Geometry: final body of the model. Coordinates: model frame, mm. Face numbers are marked on the shaded views. A direction names the side the tool comes from. Coordinates: 2 decimals unless noted, no trailing zeros. Use CSV: the item, a comma, the result in double quotes. Start each with the question number.
1. Set-up query: the marked faces 1, 2 and 3. Return all of +Z, -Z, +X, -X, +Y, -Y with unobstructed straight access to the full face (end or side cutting, diameter ignored); none if empty.
2. Material intervals for line 1 (X direction, y = -4.5, z = 0); line 2 (Z direction, x = 14.2, y = -2.75); line 3 (Y direction, x = -9, z = 9.5), sorted ascending.
3. First-contact query: P1, Ø1.6, axis at x = 1, y = 2, coming from the +Z side; P2, Ø2.5, axis at x = -4.5, y = 2, coming from the -Z side; P3, Ø1, axis at y = 1, z = 4, coming from the +X side; P4, Ø3, axis at x = -12.5, y = 8.5, coming from the -Z side. Flat tips, straight axial feed; report the tip coordinate or a pass-through.
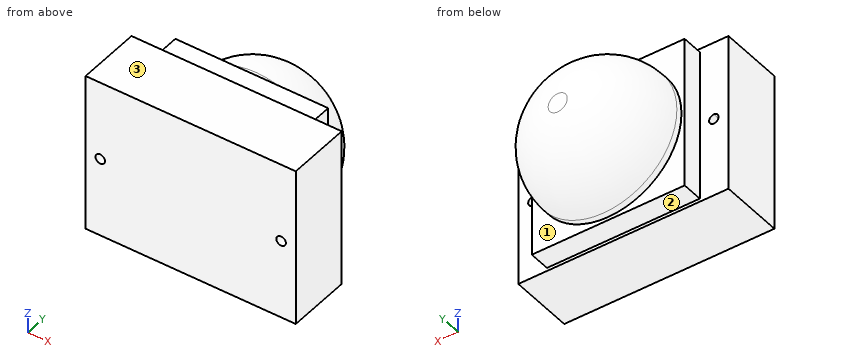
from build123d import *

# Parameters (mm, degrees)
F0_W     = 24
F0_H     = 24
F1_DEPTH = 10
F2_DEPTH = 3.3
F3_R     = 11.5
F4_DEPTH = 11
F5_R     = 10
F6_DEPTH = 10


with BuildPart() as f1:
    # F0 (on Front) → F1 (new body)
    with BuildSketch(Plane.XZ):
        with BuildLine():
            ThreePointArc((14.95, 0), (14.73033, 0.53033), (14.2, 0.75))
            ThreePointArc((14.2, 0.75), (13.66967, -0.53033), (14.95, 0))
        make_face()
        with BuildLine():
            ThreePointArc((-13.45, 0), (-13.66967, 0.53033), (-14.2, 0.75))
            ThreePointArc((-14.2, 0.75), (-14.73033, -0.53033), (-13.45, 0))
        make_face()
        Polygon((-16.5, -12.5), (16.5, -12.5), (16.5, 12.5), (14.2, 12.5), (-14.2, 12.5), (-16.5, 12.5), align=None)
        with BuildLine():
            ThreePointArc((-13.45, 0), (-14.73033, -0.53033), (-14.2, 0.75))
            ThreePointArc((-14.2, 0.75), (-13.66967, 0.53033), (-13.45, 0))
        make_face(mode=Mode.SUBTRACT)
        Rectangle(F0_W, F0_H, mode=Mode.SUBTRACT)
        with BuildLine():
            ThreePointArc((14.95, 0), (13.66967, -0.53033), (14.2, 0.75))
            ThreePointArc((14.2, 0.75), (14.73033, 0.53033), (14.95, 0))
        make_face(mode=Mode.SUBTRACT)
        Rectangle(F0_W, F0_H)
    extrude(amount=F1_DEPTH)

    # F0 (on Front) → F2 (join)
    with BuildSketch(Plane.XZ):
        Rectangle(F0_W, F0_H)
    extrude(amount=-F2_DEPTH)

    # F3 (on face) → F4 (join)
    with BuildSketch(Plane(origin=(0, 3.3, 0), x_dir=(-1, 0, 0), z_dir=(0, 1, 0))):
        Circle(F3_R)
    extrude(amount=F4_DEPTH)

    # F5
    f5_edges = [f1.edges().sort_by_distance(p)[0] for p in [
        (11.5, 14.3, 0),
    ]]
    fillet(f5_edges, radius=F5_R)

    # F0 (on Front) → F6 (cut)
    with BuildSketch(Plane.XZ):
        with BuildLine():
            ThreePointArc((14.95, 0), (14.73033, 0.53033), (14.2, 0.75))
            ThreePointArc((14.2, 0.75), (13.66967, -0.53033), (14.95, 0))
        make_face()
        with BuildLine():
            ThreePointArc((-13.45, 0), (-13.66967, 0.53033), (-14.2, 0.75))
            ThreePointArc((-14.2, 0.75), (-14.73033, -0.53033), (-13.45, 0))
        make_face()
    extrude(amount=F6_DEPTH, mode=Mode.SUBTRACT)


solid = f1.part
Results list:
1,face 1,"+Y"
1,face 2,"-Z, +X, -X, +Y"
1,face 3,"+Z, +X, -X, +Y, -Y"
2,line 1,"x = -16.5 to -14.95, -13.45 to 13.45, 14.95 to 16.5"
2,line 2,"z = -12.5 to -0.75, 0.75 to 12.5"
2,line 3,"y = -10 to 3.3"
3,P1,"stops at z = 12"
3,P2,"stops at z = -12"
3,P3,"stops at x = 12"
3,P4,"passes through"
